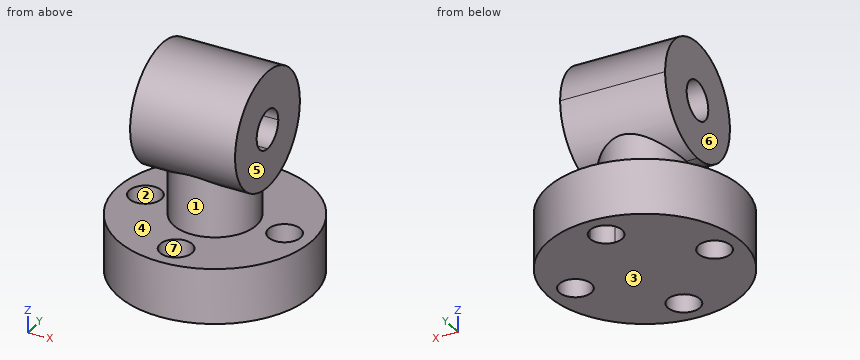
```python
from build123d import *

# Parameters (mm, degrees)
F0_R     = 11.176
F0_R_2   = 1.85
F1_DEPTH = 6.35
F2_R     = 4.7625
F3_DEPTH = 8.255
F5_DEPTH = 6.0325


with BuildPart() as f1:
    # F0 (on Top) → F1 (new body)
    with BuildSketch(Plane.XY):
        Circle(F0_R)
        with Locations((0, -8)):
            Circle(F0_R_2, mode=Mode.SUBTRACT)
        with Locations((-8, 0)):
            Circle(F0_R_2, mode=Mode.SUBTRACT)
        with Locations((8, 0)):
            Circle(F0_R_2, mode=Mode.SUBTRACT)
        with BuildLine():
            ThreePointArc((0, 6.15), (-1.308148, 9.308148), (1.85, 8))
            ThreePointArc((1.85, 8), (1.308148, 6.691852), (0, 6.15))
        make_face(mode=Mode.SUBTRACT)
    extrude(amount=F1_DEPTH)

    # F2 (on face) → F3 (join)
    with BuildSketch(Plane.XY.offset(6.35)):
        Circle(F2_R)
    extrude(amount=F3_DEPTH)

    # F4 (on Right) → F5 (join, symmetric)
    with BuildSketch(Plane.YZ):
        with BuildLine():
            ThreePointArc((6.6675, 17.78), (-4.714634, 22.494634), (0, 11.1125))
            ThreePointArc((0, 11.1125), (4.714634, 13.065366), (6.6675, 17.78))
        make_face()
        with BuildLine():
            ThreePointArc((2.2225, 17.78), (1.571545, 16.208455), (0, 15.5575))
            ThreePointArc((0, 15.5575), (-1.571545, 19.351545), (2.2225, 17.78))
        make_face(mode=Mode.SUBTRACT)
    extrude(amount=F5_DEPTH, both=True)


solid = f1.part
```
The listing builds one solid part. Answer for the finished solid, in the listing's coordinates (mm). Face numbers are marked on the shaded views. A direction names the side the tool comes from. Give positions to 0.01 mm unless a question says otherwise; leave off trailing zeros. Loops run counter-clockwise (first coordinate to the right, second up) from the corner with the lowest first, then second, coordinate; pieces in that order, holes last. Notation, with made-up numbers: (15, -37.75) - (44, -37.75) arc R14 ccw to (44, -18.75) - close; hole circle Ø6 at (-27, -1.5). An arc over 180 degrees is marked (long way). Return JSON: item names as keys, results as strings. Group by question number.
1. Find section A-A (y = 5.5). Write down the section's boundary in (x, z), then the cut area to 3 significant figures.
2. Straight lines are drawn through the part: line 1 (Z direction, x = -1.5, y = 0); line 2 (Z direction, x = -10, y = -2); line 3 (Z direction, x = -3, y = -5). For each, find the intervals that lie inside material, in ascending order. Write a range as [from, to].
3. Given pin 1 Ø1.5 at (y, z) = (3, 5) entering from -X; pin 2 Ø6.5 at (y, z) = (-1.5, 20.5) entering from +X; pin 3 Ø1 at (x, z) = (3.5, 15.5) entering from +Y, each flat-ended and moving along its own axis, determine where each tip first touches the part or whether it passes through.
4. Which of the six approach directions +Z, -Z, +X, -X, +Y, -Y give full straight-line access (tool end or side, diameter ignored) to the marked faces 4, 5, 6 and 7?
5. Find section B-B (z = 5). Write down the section's boundary in (x, y).
6. Determine the mould class of the marked faces 1, 2 and 3 for opening direction Z: pulls with the +Z half, pulls with the -Z half, needs draft (parallel to the pull), parting line crosses it, or undercut.
7. Find section C-C (x = -9). Write down the section's boundary in (y, z), then the cut area to 3 significant figures.
Verdict:
{
 "1": {"outline": "(-9.73, 0) - (9.73, 0) - (9.73, 6.35) - (-9.73, 6.35) - close; (-6.03, 14.01) - (6.03, 14.01) - (6.03, 21.55) - (-6.03, 21.55) - close", "area": "215 mm^2"},
 "2": {"line 1": "z = [0, 15.56], [20, 24.45]", "line 2": "z = [0, 6.35]", "line 3": "z = [0, 6.35], [13.37, 22.19]"},
 "3": {"pin 1": "stops at x = -10.95", "pin 2": "stops at x = 6.03", "pin 3": "stops at y = 6.43"},
 "4": {"face 4": "none", "face 5": "+Z, +X, +Y, -Y", "face 6": "+Z, -X, +Y, -Y", "face 7": "-Z"},
 "5": {"outline": "circle Ø22.35 at (0, 0); hole circle Ø3.7 at (-8, 0); hole circle Ø3.7 at (0, -8); hole (0, 6.15) arc R1.85 ccw to (1.85, 8) arc R1.85 ccw (long way) to start; hole circle Ø3.7 at (8, 0)"},
 "6": {"face 1": "undercut", "face 2": "needs draft", "face 3": "pulls with the -Z half"},
 "7": {"outline": "(-6.63, 0) - (-1.56, 0) - (-1.56, 6.35) - (-6.63, 6.35) - close; (1.56, 0) - (6.63, 0) - (6.63, 6.35) - (1.56, 6.35) - close", "area": "64.4 mm^2"}
}
